For this review, take the finished solid that the model builds, in its own axes (mm). A direction names the side the tool comes from. Round coordinates to 2 decimals unless told otherwise and drop trailing zeros. Write each loop counter-clockwise with the first axis right and the second up, starting at its lowest first coordinate (ties: lowest second). Pieces come first, ordered by that corner, then holes. Notation, with made-up numbers: (-10.5, 81.25) -> (40.5, 81.25) arc R23 ccw to (40.5, 96.25) -> close; hole circle Ø10 at (31, 27). An arc over 180 degrees is marked (long way). Answer as CSV lines item,"result". Start each with the question number.
Item 1: For pin 1 Ø4 at (x, y) = (9, 0) entering from +Z; pin 2 Ø6 at (y, z) = (1, 4) entering from +X; pin 3 Ø3 at (x, y) = (-2, -0.5) entering from +Z; pin 4 Ø1 at (x, y) = (3.5, 0.5) entering from +Z, all flat-tipped, find the tip position at first contact; note any pin that passes through.
Item 2: Mouldability with a two-part tool opening along Y and no side actions: class faces 3 (the cylindrical face through (-10.5, 0.07, 1.73)), 4 (the flat face through (3.2, 4.3, 3.5)), 5 (the cylindrical face through (2.4, -4.5, -1)) as +Y half, -Y half, draft (parallel to the pull), parting line (faces both ways), or undercut.
Item 3: Take a section at D-D on x = 0. Give the boundary of the cut face in (y, z).
Item 4: Machinability: for faces 1 (the cylindrical face through (2.4, -4.5, 6)), 2 (the flat face through (0, -6.3, 2)), which of the approach directions +Z, -Z, +X, -X, +Y, -Y give a long, thin tool a straight path to every point of the face, cutting with its end or side? Answer none if there is none.
Item 5: Take a section at A-A on x = 9. Give the boundary of the cut face in (y, z), then the cut area to 3 significant figures.
Item 6: Take a section at C-C on y = 0. Give the boundary of the cut face in (x, z).
Item 7: Wall thickness on probe 1 along X at (y, z) = (0.5, 0.25); probe 2 along Y at (x, z) = (9, 2.8); probe 3 along Z at (x, y) = (-5.25, -1.5): over which ranges is each line inside the solid? List them lowest first. Write a range as from..to.
Item 8: Take a section at B-B on z = 1.5. Give the boundary of the cut face in (x, y), then the cut area to 3 significant figures.
```python
from build123d import *

# Parameters (mm, degrees)
SKICA1_R                     = 1.5
P_IDAT_VYSUNUT_M1_DEPTH      = 3.5
P_IDAT_VYSUNUT_M2_DEPTH      = 5
P_IDAT_VYSUNUT_M2_DEPTH_BACK = 5.5
SKICA2_R                     = 5.1
SKICA3_R                     = 4
ODEBRAT_VYSUNUT_M1_DEPTH     = 10.5
ZKOSEN_1_SIZE                = 0.5


with BuildPart() as part:
    # Skica1 → Přidat vysunutím1 (new body)
    with BuildSketch(Plane.XY):
        with BuildLine():
            Line((-11.939849245, 6.3), (11.939849245, 6.3))
            ThreePointArc((11.939849245, 6.3), (13.5, 0), (11.939849245, -6.3))
            Line((11.939849245, -6.3), (-11.939849245, -6.3))
            ThreePointArc((-11.939849245, -6.3), (-13.5, 0), (-11.939849245, 6.3))
        make_face()
        with Locations((-9, 0)):
            Circle(SKICA1_R, mode=Mode.SUBTRACT)
        with Locations((9, 0)):
            Circle(SKICA1_R, mode=Mode.SUBTRACT)
    extrude(amount=P_IDAT_VYSUNUT_M1_DEPTH)

    # Skica2 → Přidat vysunutím2 (add, two sides: drawn at the far end of the back side and taken through both)
    with BuildSketch(Plane.XY.offset(3.5).offset(-P_IDAT_VYSUNUT_M2_DEPTH_BACK)):
        Circle(SKICA2_R)
    extrude(amount=P_IDAT_VYSUNUT_M2_DEPTH + P_IDAT_VYSUNUT_M2_DEPTH_BACK)

    # Skica3 → Odebrat vysunutím1 (cut)
    with BuildSketch(Plane.XY.offset(8.5)):
        Circle(SKICA3_R)
    extrude(amount=-ODEBRAT_VYSUNUT_M1_DEPTH, mode=Mode.SUBTRACT)

    # Zkosení1
    zkosen_1_edges = [part.edges().sort_by_distance(p)[0] for p in [
        (-4, 0, 8.5),
        (-4, 0, -2),
    ]]
    chamfer(zkosen_1_edges, length=ZKOSEN_1_SIZE)


solid = part.part
```
Output values:
1,pin 1,"stops at z = 3.5"
1,pin 2,"stops at x = 13.5"
1,pin 3,"passes through"
1,pin 4,"stops at z = 8.04"
2,face 3,"undercut"
2,face 4,"draft"
2,face 5,"parting line"
3,outline,"(-6.3, 0) -> (-5.1, 0) -> (-5.1, -2) -> (-4.5, -2) -> (-4, -1.5) -> (-4, 8) -> (-4.5, 8.5) -> (-5.1, 8.5) -> (-5.1, 3.5) -> (-6.3, 3.5) -> close; (4, -1.5) -> (4.5, -2) -> (5.1, -2) -> (5.1, 0) -> (6.3, 0) -> (6.3, 3.5) -> (5.1, 3.5) -> (5.1, 8.5) -> (4.5, 8.5) -> (4, 8) -> close"
4,face 1,"+Z"
4,face 2,"+Z, -Z, +X, -X, -Y"
5,outline,"(-6.3, 0) -> (-1.5, 0) -> (-1.5, 3.5) -> (-6.3, 3.5) -> close; (1.5, 0) -> (6.3, 0) -> (6.3, 3.5) -> (1.5, 3.5) -> close"
5,area,"33.6 mm^2"
6,outline,"(-13.5, 0) -> (-10.5, 0) -> (-10.5, 3.5) -> (-13.5, 3.5) -> close; (-7.5, 0) -> (-5.1, 0) -> (-5.1, -2) -> (-4.5, -2) -> (-4, -1.5) -> (-4, 8) -> (-4.5, 8.5) -> (-5.1, 8.5) -> (-5.1, 3.5) -> (-7.5, 3.5) -> close; (4, -1.5) -> (4.5, -2) -> (5.1, -2) -> (5.1, 0) -> (7.5, 0) -> (7.5, 3.5) -> (5.1, 3.5) -> (5.1, 8.5) -> (4.5, 8.5) -> (4, 8) -> close; (10.5, 0) -> (13.5, 0) -> (13.5, 3.5) -> (10.5, 3.5) -> close"
7,probe 1,"x = -13.49..-10.41, -7.59..-3.97, 3.97..7.59, 10.41..13.49"
7,probe 2,"y = -6.3..-1.5, 1.5..6.3"
7,probe 3,"z = 0..3.5"
8,outline,"(-11.94, -6.3) -> (11.94, -6.3) arc R13.5 ccw to (11.94, 6.3) -> (-11.94, 6.3) arc R13.5 ccw to start; hole circle Ø3 at (-9, 0); hole circle Ø8 at (0, 0); hole circle Ø3 at (9, 0)"
8,area,"263 mm^2"
